```python
from build123d import *

# Parameters (mm, degrees)
F1_DEPTH = 4.2


with BuildPart() as f1:
    # F0 (on Top) → F1 (new body)
    with BuildSketch(Plane.XY):
        with BuildLine():
            Line((-21.753184, 26.967989), (-21.753184, -38.291566))
            Line((-21.753184, -38.291566), (-15.49542, -38.291566))
            Line((-15.49542, -38.291566), (-15.49542, 26.967989))
            Line((-15.49542, 26.967989), (-11.718347, 26.967989))
            Line((-11.718347, 26.967989), (-11.718347, 25.370423))
            Line((-11.718347, 25.370423), (-7.504017, 25.370423))
            Line((-7.504017, 25.370423), (-7.504017, 31.270303))
            Line((-7.504017, 31.270303), (-11.718347, 31.270303))
            Line((-11.718347, 31.270303), (-11.718347, 29.373912))
            Line((-11.718347, 29.373912), (-21.753184, 29.373912))
            ThreePointArc((-21.753184, 29.373912), (-31.188051, 26.714196), (-37.844583, 19.518269))
            ThreePointArc((-37.844583, 19.518269), (-30.619292, 25.015211), (-21.753184, 26.967989))
        make_face()
    extrude(amount=F1_DEPTH)


solid = f1.part
```
The listing builds one solid part. Answer for the finished solid, in the listing's coordinates (mm). A direction names the side the tool comes from. Give positions to 0.01 mm unless a question says otherwise; leave off trailing zeros. Order: outer loops, then holes, each group sorted by start corner. A loop starts at its lowest first (then second) coordinate and runs counter-clockwise, first axis right, second up. Notation, with made-up numbers: M 30.5,-26.75 L 50.5,-26.75 A19 cw 50.5,-21.75 Z; hole C 35,9.25 d5. An arc over 180 degrees is marked long. Put each result on its own line as item: value. Start each with the question number.
Item 1: Flat-ended cylindrical pins translate along their axes: P1, Ø2, axis at x = -9.5, z = 2.5, coming from the -Y side; P2, Ø1, axis at y = -10.5, z = 1.5, coming from the -X side; P3, Ø0.5, axis at y = 26, z = 1.5, coming from the -X side. Find the tip coordinate at first contact, or state that the pin passes through.
Item 2: For a pull along X with two mould halves and no side action, classify faces 1 (the face through (-11.718, 26, 2)), 2 (the face through (-17, 29.374, 2)), 3 (the face through (-11.718, 30, 2)) as +X half, -X half, draft (parallel to the pull), parting line (faces both ways), or undercut.
Item 3: Which of the six approach directions +Z, -Z, +X, -X, +Y, -Y give full straight-line access (tool end or side, diameter ignored) to faces 4 (the face through (-10, 25.37, 2)), 5 (the face through (-30.74, 24.96, 2.07)), 6 (the face through (-18, -1, 0))?
Item 4: Find the intervals of material crossed by line 1 along X through (y, z) = (-25.5, 0.35); line 2 along Y through (x, z) = (-17, 1.6); line 3 along Y through (x, z) = (-15, 0.35), in increasing order.
Item 5: The part is cut by section A-A, the plane z = 2.4. Determine the outline of the cut face in (x, y), and give its area (3 significant figures).
Item 6: The part is cut by section B-B, the plane y = 16. Determine the outline of the cut face in (x, z).
Item 7: The part is cut by section C-C, the plane x = -20. Determine the outline of the cut face in (y, z).
Answer key:
1. P1: stops at y = 25.37
1. P2: stops at x = -21.75
1. P3: stops at x = -32.61
2. face 1: undercut
2. face 2: draft
2. face 3: -X half
3. face 4: +Z, -Z, +X, -Y
3. face 5: +Z, -Z, -Y
3. face 6: -Z, +X, -X, +Y, -Y
4. line 1: x = -21.75 to -15.5
4. line 2: y = -38.29 to 29.37
4. line 3: y = 26.97 to 29.37
5. outline: M -37.84,19.52 A21.1 cw -21.75,26.97 L -21.75,-38.29 L -15.5,-38.29 L -15.5,26.97 L -11.72,26.97 L -11.72,25.37 L -7.5,25.37 L -7.5,31.27 L -11.72,31.27 L -11.72,29.37 L -21.75,29.37 A18.06 ccw Z
5. area: 487 mm²
6. outline: M -21.75,0 L -15.5,0 L -15.5,4.2 L -21.75,4.2 Z
7. outline: M -38.29,0 L 29.37,0 L 29.37,4.2 L -38.29,4.2 Z
